Check sheet for the modelled part. Datum: model origin and axes. Units: mm. A direction names the side the tool comes from. Coordinates: 2 decimals unless noted, no trailing zeros. Order: outer loops, then holes, each group sorted by start corner. A loop starts at its lowest first (then second) coordinate and runs counter-clockwise, first axis right, second up.
1. Cross-section at C-C (y = 0). Enter the section's corners in (x, z).
2. Cross-section at D-D (x = -2). Enter the section's corners in (y, z).
3. Cross-section at A-A (x = 1.75). Enter the section's corners in (y, z).
4. Thickness scan on line 1 (Y direction, x = 1.75, z = 1.05); line 2 (Y direction, x = -1.25, z = 0.15); line 3 (X direction, y = -0.75, z = 0.2). Record the ranges inside material, lowest first.
5. Draft check along X on faces 3 (the cylindrical face through (1.27, -0.97, 0.78)), 4 (the cylindrical face through (-0.285, -4.201, 0.783)), 5 (the flat face through (2, -1, 0)). Enter one of: released by +X, released by -X, zero draft, split by the parting line, or undercut.
6. Cross-section at B-B (z = 0.75). Enter the section's corners in (x, y).
7. Set-up check for faces 1 (the flat face through (0, 3.9, 1)), 2 (the flat face through (-2, -3.9, 1)): record each of +Z, -Z, +X, -X, +Y, -Y from which the full face is reachable in a straight line by a thin tool's end or side.
8. Gauge pin test, flat end, axial feed: pin 1 Ø1 at (x, y) = (1.5, -5) entering from -Z. Record the tip position at first contact, or that the pin passes through.
```python
from build123d import *

# Parameters (mm, degrees)
SKETCH1_R           = 0.75
SKETCH1_R_2         = 1.6
BOSS_EXTRUDE1_DEPTH = 1.5875


with BuildPart() as part:
    # Sketch1 → Boss-Extrude1 (new body)
    with BuildSketch(Plane(origin=(0, 0, 0), x_dir=(-1, 0, 0), z_dir=(0, 0, -1))):
        with BuildLine():
            Line((3.5, -3.9), (3.5, 3.9))
            Line((3.5, 3.9), (-3.5, 3.9))
            Line((-3.5, 3.9), (-3.5, -5.18125))
            ThreePointArc((-3.5, -5.18125), (-3.207106781, -5.888356781), (-2.5, -6.18125))
            Line((-2.5, -6.18125), (-1, -6.18125))
            ThreePointArc((-1, -6.18125), (-0.292893219, -5.888356781), (0, -5.18125))
            Line((0, -5.18125), (0, -4.9))
            ThreePointArc((0, -4.9), (0.292893219, -4.192893219), (1, -3.9))
            Line((1, -3.9), (3.5, -3.9))
        make_face()
        with Locations((-1.75, -4.7)):
            Circle(SKETCH1_R, mode=Mode.SUBTRACT)
        Circle(SKETCH1_R_2, mode=Mode.SUBTRACT)
    extrude(amount=-BOSS_EXTRUDE1_DEPTH)


solid = part.part
```
Data:
1. outline: (-3.5, 0) - (-1.6, 0) - (-1.6, 1.59) - (-3.5, 1.59) - close; (1.6, 0) - (3.5, 0) - (3.5, 1.59) - (1.6, 1.59) - close
2. outline: (-3.9, 0) - (3.9, 0) - (3.9, 1.59) - (-3.9, 1.59) - close
3. outline: (-6.18, 0) - (-5.45, 0) - (-5.45, 1.59) - (-6.18, 1.59) - close; (-3.95, 0) - (3.9, 0) - (3.9, 1.59) - (-3.95, 1.59) - close
4. line 1: y = -6.18 to -5.45, -3.95 to 3.9
4. line 2: y = -3.9 to -1, 1 to 3.9
4. line 3: x = -3.5 to -1.41, 1.41 to 3.5
5. face 3: undercut
5. face 4: released by -X
5. face 5: zero draft
6. outline: (-3.5, -3.9) - (-1, -3.9) arc R1 cw to (0, -4.9) - (0, -5.18) arc R1 ccw to (1, -6.18) - (2.5, -6.18) arc R1 ccw to (3.5, -5.18) - (3.5, 3.9) - (-3.5, 3.9) - close; hole circle Ø3.2 at (0, 0); hole circle Ø1.5 at (1.75, -4.7)
7. face 1: +Z, -Z, +X, -X, +Y
7. face 2: +Z, -Z, -X, -Y
8. pin 1: stops at z = 0
